```python
from build123d import *

# Parameters (mm, degrees)
F1_DEPTH = 10
F2_DEPTH = 5
F3_R     = 4
F4_DEPTH = 7
F5_R     = 1.448528


with BuildPart() as f1:
    # F0 (on Top) → F1 (new body)
    with BuildSketch(Plane.XY):
        Polygon((12.990381, -22.5), (12.990381, 22.5), (-25.980762, 0), align=None)
        Polygon((-17.320508, 0), (8.660254, 15), (8.660254, -15), align=None, mode=Mode.SUBTRACT)
    extrude(amount=F1_DEPTH)

    # F0 (on Top) → F2 (join)
    with BuildSketch(Plane.XY):
        Polygon((12.990381, -22.5), (12.990381, 22.5), (-25.980762, 0), align=None)
        Polygon((-17.320508, 0), (8.660254, 15), (8.660254, -15), align=None, mode=Mode.SUBTRACT)
        Polygon((8.660254, -15), (8.660254, 15), (-17.320508, 0), align=None)
    extrude(amount=-F2_DEPTH)

    # F3 (on face) → F4 (join)
    with BuildSketch(Plane(origin=(0, 0, -5), x_dir=(1, 0, 0), z_dir=(0, 0, -1))):
        Circle(F3_R)
    extrude(amount=F4_DEPTH)

    # F5
    f5_edges = [f1.edges().sort_by_distance(p)[0] for p in [
        (4, 0, -8.5),
        (-4, 0, -5),
        (-4, 0, -12),
    ]]
    fillet(f5_edges, radius=F5_R)


solid = f1.part
```
Model file for the job. Use its own axes, mm. A direction names the side the tool comes from. Coordinates: 2 decimals unless noted, no trailing zeros. Loops run counter-clockwise (first coordinate to the right, second up) from the corner with the lowest first, then second, coordinate; pieces in that order, holes last. Notation, with made-up numbers: (14, 24.25) - (18, 24.25) arc R22 ccw to (18, 39.25) - close; hole circle Ø6 at (78.5, 69.5). An arc over 180 degrees is marked (long way). Answer as a JSON object with one key per item and string values. Group by question number.
(1) Cut at D-D (z = -10). Give the cut face in (x, y), then the cut area to 3 significant figures.
(2) Two-plate mould, pull along Y, no slides. Class faces 1 (the face through (-6.22, 11.41, 2.61)), 2 (the face through (-6.77, -11.09, 2.61)), 3 (the face through (-4.148, -7.605, 4.93)): released by +Y, released by -Y, zero draft, split by the parting line, or undercut.
(3) Cut at C-C (y = 7). Give the cut face in (x, z).
(4) Cut at A-A (x = 0). Give the cut face in (y, z), then the cut area to 3 significant figures.
(5) Probe line 1 along Z through (x, y) = (8.5, 0); line 2 along Z through (x, y) = (-15.5, -2); line 3 along Y through (x, z) = (-1.5, 6). List the from-to ranges inside material, lowest first.
(6) Flat gauge pins, fed straight in: pin 1 (6 mm diameter, centred on x = 6, z = 1.5, fed in from -Y); pin 2 (4 mm diameter, centred on y = 13.5, z = 0, fed in from -X); pin 3 (4 mm diameter, centred on x = -15.5, z = -5.5, fed in from -Y). Where does each tip first touch, or does it go through?
(7) Tool access for faces 4 (the face through (-0.867, 3.905, -8.471)), 5 (the face through (-4, -8, 10)), 6 (the face through (-4.5, 7.4, 4.9)): list every direction of +Z, -Z, +X, -X, +Y, -Y with a clear straight run to the whole face (end or side of a thin tool).
(8) Cut at B-B (z = 5.5). Give the cut face in (x, y).
Geometry says:
{
 "1": {"outline": "circle Ø8 at (0, 0)", "area": "50.3 mm^2"},
 "2": {"face 1": "released by +Y", "face 2": "released by -Y", "face 3": "undercut"},
 "3": {"outline": "(-13.86, -5) - (12.99, -5) - (12.99, 10) - (8.66, 10) - (8.66, 0) - (-5.2, 0) - (-5.2, 10) - (-13.86, 10) - close"},
 "4": {"outline": "(-15, -5) - (-5.45, -5) arc R1.45 cw to (-4, -6.45) - (-4, -10.55) arc R1.45 ccw to (-2.55, -12) - (2.55, -12) arc R1.45 ccw to (4, -10.55) - (4, -6.45) arc R1.45 cw to (5.45, -5) - (15, -5) - (15, 10) - (10, 10) - (10, 0) - (-10, 0) - (-10, 10) - (-15, 10) - close", "area": "306 mm^2"},
 "5": {"line 1": "z = -5 to 0", "line 2": "z = -5 to 10", "line 3": "y = -14.13 to -9.13, 9.13 to 14.13"},
 "6": {"pin 1": "stops at y = -20.2", "pin 2": "stops at x = -6.06", "pin 3": "stops at y = -7.17"},
 "7": {"face 4": "-Z", "face 5": "+Z, +X, -X, +Y, -Y", "face 6": "+Z"},
 "8": {"outline": "(-25.98, 0) - (12.99, -22.5) - (12.99, 22.5) - close; hole (-17.32, 0) - (8.66, -15) - (8.66, 15) - close"}
}
